```python
from build123d import *

# Parameters (mm, degrees)
F0_W     = 150
F0_H     = 100
F1_DEPTH = 1
F2_W     = 30
F2_H     = 15
F2_W_2   = 80
F3_DEPTH = 1.001
F4_W     = 1
F4_H     = 20
F4_W_2   = 20
F4_H_2   = 1
F5_DEPTH = 8
F6_W     = 2
F6_H     = 50
F6_W_2   = 40
F6_H_2   = 2
F6_W_3   = 30
F6_H_3   = 43
F7_DEPTH = 9.001


with BuildPart() as f1:
    # F0 (on Top) → F1 (new body)
    with BuildSketch(Plane.XY):
        Rectangle(F0_W, F0_H)
    extrude(amount=F1_DEPTH)

    # F2 (on face) → F3 (cut, through all)
    with BuildSketch(Plane.XY.offset(1)):
        with Locations((-60, 42.5)):
            Rectangle(F2_W, F2_H)
        with Locations((15, 42.5)):
            Rectangle(F2_W_2, F2_H)
    extrude(amount=-F3_DEPTH, mode=Mode.SUBTRACT)

    # F4 (on face) → F5 (join)
    with BuildSketch(Plane(origin=(0, 0, 0), x_dir=(1, 0, 0), z_dir=(0, 0, -1))):
        with Locations((-74.5, -25)):
            Rectangle(F4_W, F4_H)
        with Locations((-35, -49.5)):
            Rectangle(F4_W_2, F4_H_2)
        with Locations((65, -49.5)):
            Rectangle(F4_W_2, F4_H_2)
        with Locations((-74.5, 40)):
            Rectangle(F4_W, F4_H)
    extrude(amount=F5_DEPTH)

    # F6 (on face) → F7 (cut, through all)
    with BuildSketch(Plane.XY.offset(1)):
        with Locations((-64, -10)):
            Rectangle(F6_W, F6_H)
        with Locations((-28, 24)):
            Rectangle(F6_W_2, F6_H_2)
        with Locations((40, 24)):
            Rectangle(F6_W_2, F6_H_2)
        with Locations((-33, -13.5)):
            Rectangle(F6_W_3, F6_H_3)
        with Locations((7, -13.5)):
            Rectangle(F6_W_3, F6_H_3)
        with Locations((47, -13.5)):
            Rectangle(F6_W_3, F6_H_3)
    extrude(amount=-F7_DEPTH, mode=Mode.SUBTRACT)


solid = f1.part
```
Geometry check sheet. Reference: the model listing, model coordinates, mm. A direction names the side the tool comes from. Give positions to 0.01 mm unless a question says otherwise; leave off trailing zeros. Write each loop counter-clockwise with the first axis right and the second up, starting at its lowest first coordinate (ties: lowest second). Pieces come first, ordered by that corner, then holes. Notation, with made-up numbers: (-30, -34) - (-7, -34) arc R20 cw to (-7, 3) - close; hole circle Ø3 at (-31.75, 46.25). An arc over 180 degrees is marked (long way). Use a Markdown table: item, result.
Q1. Set-up check for faces 5 (the face through (55, 45.2, 0.2)), 6 (the face through (-74, -40, -4)), 7 (the face through (-35, 50, -4)), 8 (the face through (-63.4, 35, 0.2)), 9 (the face through (65, 49, -4)): record each of +Z, -Z, +X, -X, +Y, -Y from which the full face is reachable in a straight line by a thin tool's end or side.
Computed:
| item | result |
|---|---|
| face 5 | +Z, -Z, +Y |
| face 6 | -Z, +X, +Y, -Y |
| face 7 | +Z, -Z, +X, -X, +Y |
| face 8 | +Z, -Z, -X, +Y |
| face 9 | -Z, +X, -X, -Y |
Q2. Draft check along X on faces 1 (the face through (-25, 45.2, 0.2)), 2 (the face through (-35, 49, -4)), 3 (the face through (-45, 45.2, 0.2)), 4 (the face through (-74, 25, -4)). Enter one of: pulls with the +X half, pulls with the -X half, needs draft (parallel to the pull), parting line crosses it, or undercut.
Computed:
| item | result |
|---|---|
| face 1 | undercut |
| face 2 | needs draft |
| face 3 | pulls with the -X half |
| face 4 | pulls with the +X half |
Q3. Section check A-A, the plane x = 24. Enter the section's corners in (y, z), then the cut area to 3 significant figures.
Computed:
| item | result |
|---|---|
| outline | (-50, 0) - (23, 0) - (23, 1) - (-50, 1) - close; (25, 0) - (35, 0) - (35, 1) - (25, 1) - close |
| area | 83.0 mm² |
Q4. Go/stop test with flat-tipped pins: P1, Ø1.1, axis at x = 39.5, z = 0.5, coming from the +Y side; P2, Ø8, axis at x = 18, y = -34, coming from the -Z side; P3, Ø4, axis at y = 27.5, z = -3.5, coming from the +X side. Record where each tip stops, or that it passes through.
Computed:
| item | result |
|---|---|
| P1 | stops at y = 35 |
| P2 | stops at z = 0 |
| P3 | stops at x = -74 |
Q5. Section check D-D, the plane x = 46.5. Enter the section's corners in (y, z).
Computed:
| item | result |
|---|---|
| outline | (-50, 0) - (-35, 0) - (-35, 1) - (-50, 1) - close; (8, 0) - (23, 0) - (23, 1) - (8, 1) - close; (25, 0) - (35, 0) - (35, 1) - (25, 1) - close |
Q6. Section check C-C, the plane z = -2.75. Enter the section's corners in (x, y).
Computed:
| item | result |
|---|---|
| outline | (-75, -50) - (-74, -50) - (-74, -30) - (-75, -30) - close; (-75, 15) - (-74, 15) - (-74, 35) - (-75, 35) - close; (-45, 49) - (-25, 49) - (-25, 50) - (-45, 50) - close; (55, 49) - (75, 49) - (75, 50) - (55, 50) - close |
Q7. Section check B-B, the plane y = 37. Enter the section's corners in (x, z), then the cut area to 3 significant figures.
Computed:
| item | result |
|---|---|
| outline | (-45, 0) - (-25, 0) - (-25, 1) - (-45, 1) - close; (55, 0) - (75, 0) - (75, 1) - (55, 1) - close |
| area | 40.0 mm² |
Q8. Thickness scan on L1, parallel to Y at x = -34.5, z = 0.5; L2, parallel to Y at x = 17, z = 0.75; L3, parallel to Z at x = 27, y = 29.5. Record the ranges inside material, lowest first. Write a range as [from, to].
Computed:
| item | result |
|---|---|
| L1 | y = [-50, -35], [8, 23], [25, 50] |
| L2 | y = [-50, -35], [8, 35] |
| L3 | z = [0, 1] |
